from build123d import *

# Parameters (mm, degrees)
SKETCH1_R           = 2.2098
BOSS_EXTRUDE1_DEPTH = 3.175
SKETCH2_R           = 3.1623
CUT_EXTRUDE3_DEPTH  = 1.27
SKETCH3_R           = 2.2098
SKETCH3_R_2         = 5.08
BOSS_EXTRUDE2_DEPTH = 2.159


with BuildPart() as part:
    # Sketch1 → Boss-Extrude1 (new body)
    with BuildSketch(Plane.XY):
        with BuildLine():
            Line((-50.8, -31.75), (50.8, -31.75))
            ThreePointArc((50.8, -31.75), (55.290128061, -29.890128061), (57.15, -25.4))
            Line((57.15, -25.4), (57.15, 25.4))
            ThreePointArc((57.15, 25.4), (55.290128061, 29.890128061), (50.8, 31.75))
            Line((50.8, 31.75), (-50.8, 31.75))
            ThreePointArc((-50.8, 31.75), (-55.290128061, 29.890128061), (-57.15, 25.4))
            Line((-57.15, 25.4), (-57.15, -25.4))
            ThreePointArc((-57.15, -25.4), (-55.290128061, -29.890128061), (-50.8, -31.75))
        make_face()
        with Locations((-50.8, -25.4)):
            Circle(SKETCH1_R, mode=Mode.SUBTRACT)
        with Locations((-38.1, -25.4)):
            Circle(SKETCH1_R, mode=Mode.SUBTRACT)
        with Locations(Location((-50.8, 25.4, 0), (0, 0, 180))):
            Circle(SKETCH1_R, mode=Mode.SUBTRACT)
        with Locations(Location((-38.1, 25.4, 0), (0, 0, 180))):
            Circle(SKETCH1_R, mode=Mode.SUBTRACT)
        with Locations((50.8, 25.4)):
            Circle(SKETCH1_R, mode=Mode.SUBTRACT)
        with Locations((38.1, 25.4)):
            Circle(SKETCH1_R, mode=Mode.SUBTRACT)
        with Locations(Location((50.8, -25.4, 0), (0, 0, 180))):
            Circle(SKETCH1_R, mode=Mode.SUBTRACT)
        with Locations(Location((38.1, -25.4, 0), (0, 0, 180))):
            Circle(SKETCH1_R, mode=Mode.SUBTRACT)
    extrude(amount=-BOSS_EXTRUDE1_DEPTH)

    # Sketch2 → Cut-Extrude3 (cut)
    with BuildSketch(Plane.XY):
        with BuildLine():
            Line((50.8, 30.7975), (-50.8, 30.7975))
            ThreePointArc((-50.8, 30.7975), (-54.616608851, 29.216608851), (-56.1975, 25.4))
            Line((-56.1975, 25.4), (-56.1975, -25.4))
            ThreePointArc((-56.1975, -25.4), (-54.616608851, -29.216608851), (-50.8, -30.7975))
            Line((-50.8, -30.7975), (50.8, -30.7975))
            ThreePointArc((50.8, -30.7975), (54.616608851, -29.216608851), (56.1975, -25.4))
            Line((56.1975, -25.4), (56.1975, 25.4))
            ThreePointArc((56.1975, 25.4), (54.616608851, 29.216608851), (50.8, 30.7975))
        make_face()
        with Locations((38.1, 25.4)):
            Circle(SKETCH2_R, mode=Mode.SUBTRACT)
        with Locations((50.8, 25.4)):
            Circle(SKETCH2_R, mode=Mode.SUBTRACT)
        with Locations((50.8, -25.4)):
            Circle(SKETCH2_R, mode=Mode.SUBTRACT)
        with Locations((38.1, -25.4)):
            Circle(SKETCH2_R, mode=Mode.SUBTRACT)
        with Locations((-38.1, -25.4)):
            Circle(SKETCH2_R, mode=Mode.SUBTRACT)
        with Locations((-50.8, -25.4)):
            Circle(SKETCH2_R, mode=Mode.SUBTRACT)
        with Locations((-38.1, 25.4)):
            Circle(SKETCH2_R, mode=Mode.SUBTRACT)
        with Locations((-50.8, 25.4)):
            Circle(SKETCH2_R, mode=Mode.SUBTRACT)
    extrude(amount=-CUT_EXTRUDE3_DEPTH, mode=Mode.SUBTRACT)

    # Sketch3 → Boss-Extrude2 (add)
    with BuildSketch(Plane(origin=(0, 0, -3.175), x_dir=(-1, 0, 0), z_dir=(0, 0, -1))):
        with BuildLine():
            Line((-57.15, 25.4), (-57.15, -25.4))
            ThreePointArc((-57.15, -25.4), (-55.290128061, -29.890128061), (-50.8, -31.75))
            Line((-50.8, -31.75), (50.8, -31.75))
            ThreePointArc((50.8, -31.75), (55.290128061, -29.890128061), (57.15, -25.4))
            Line((57.15, -25.4), (57.15, 25.4))
            ThreePointArc((57.15, 25.4), (55.290128061, 29.890128061), (50.8, 31.75))
            Line((50.8, 31.75), (-50.8, 31.75))
            ThreePointArc((-50.8, 31.75), (-55.290128061, 29.890128061), (-57.15, 25.4))
        make_face()
        with Locations((-50.8, -25.4)):
            Circle(SKETCH3_R, mode=Mode.SUBTRACT)
        with Locations((-38.1, -25.4)):
            Circle(SKETCH3_R, mode=Mode.SUBTRACT)
        with Locations(Location((38.1, -25.4, 0), (0, 0, 180))):
            Circle(SKETCH3_R, mode=Mode.SUBTRACT)
        with Locations(Location((50.8, -25.4, 0), (0, 0, 180))):
            Circle(SKETCH3_R, mode=Mode.SUBTRACT)
        with Locations((50.8, 25.4)):
            Circle(SKETCH3_R, mode=Mode.SUBTRACT)
        with Locations((38.1, 25.4)):
            Circle(SKETCH3_R, mode=Mode.SUBTRACT)
        with Locations(Location((-38.1, 25.4, 0), (0, 0, 180))):
            Circle(SKETCH3_R, mode=Mode.SUBTRACT)
        with Locations(Location((-50.8, 25.4, 0), (0, 0, 180))):
            Circle(SKETCH3_R, mode=Mode.SUBTRACT)
        Circle(SKETCH3_R_2, mode=Mode.SUBTRACT)
        with Locations((38.1, 0)):
            Circle(SKETCH3_R_2, mode=Mode.SUBTRACT)
        with Locations((-38.1, 0)):
            Circle(SKETCH3_R_2, mode=Mode.SUBTRACT)
    extrude(amount=BOSS_EXTRUDE2_DEPTH)


solid = part.part
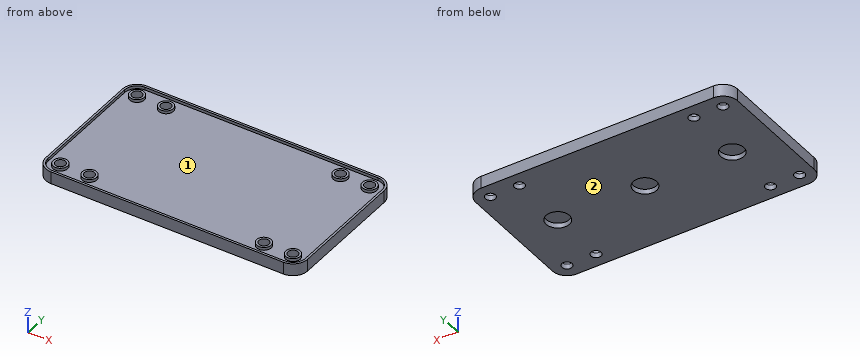
Verification items for the finished model (mm, model axes). Face numbers are marked on the shaded views. Coordinates: 2 decimals unless noted, no trailing zeros. Order: outer loops, then holes, each group sorted by start corner. A loop starts at its lowest first (then second) coordinate and runs counter-clockwise, first axis right, second up.
1. Go/stop test with flat-tipped pins: pin 1 Ø5 at (x, y) = (1.5, -1) entering from -Z (3 decimals); pin 2 Ø8 at (x, y) = (0, 0) entering from +Z. Record where each tip stops, or that it passes through.
Results found:
pin 1: stops at z = -3.175
pin 2: stops at z = -1.27
2. Sectioned sample at A-A, the plane x = -38.1. Give the number of separate pieces and of enclosed holes in the cut face, and give its area (3 significant figures).
Results found:
separate pieces: 3
enclosed holes: 0
area: 207 mm2
3. Scan lines: line 1 (Y direction, x = 38.1, z = -4.8); line 2 (Y direction, x = -38.1, z = -1.9); line 3 (X direction, y = 25.4, z = -3.75). Record each from-to range of solid material in increasing order.
Results found:
line 1: y = -31.75 to -27.61, -23.19 to -5.08, 5.08 to 23.19, 27.61 to 31.75
line 2: y = -31.75 to -27.61, -23.19 to 23.19, 27.61 to 31.75
line 3: x = -57.15 to -53.01, -48.59 to -40.31, -35.89 to 35.89, 40.31 to 48.59, 53.01 to 57.15
4. Release check for a two-part mould opening along Y. For the marked faces 1 and 2 record: +Y half, -Y half, draft (parallel to the pull), parting line (faces both ways), or undercut.
Results found:
face 1: undercut
face 2: draft
5. Sectioned sample at D-D, the plane y = -15. Record the cut outline in (x, z).
Results found:
outline: (-57.15, -5.33) - (57.15, -5.33) - (57.15, 0) - (56.2, 0) - (56.2, -1.27) - (-56.2, -1.27) - (-56.2, 0) - (-57.15, 0) - close
